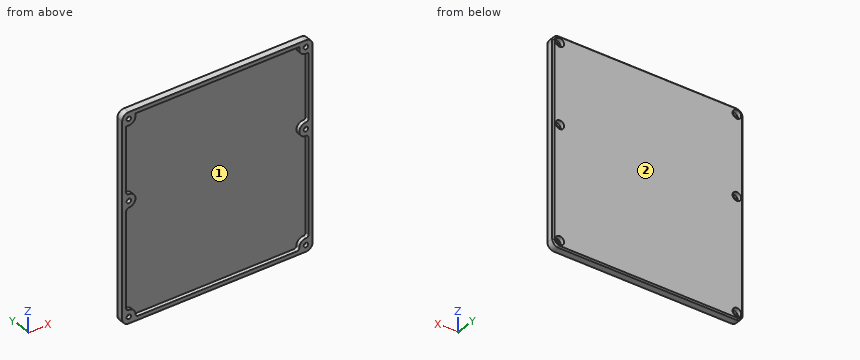
```python
from build123d import *

# Parameters (mm, degrees)
SKETCH_1_W                   = 144
SKETCH_1_H                   = 157
EXTRUDE_1_DEPTH              = 6
FILLET_1_R                   = 5
SHELL_1_T                    = -3
EXTRUDE_2_DEPTH              = 6
HOLE_WIZARD_M3_1_D           = 3.4
HOLE_WIZARD_M3_1_CBORE_D     = 6.5
HOLE_WIZARD_M3_1_CBORE_DEPTH = 3.4
CHAMFER_1_SIZE               = 1
FILLET_4_R                   = 2


with BuildPart() as part:
    # 草图1 → 凸台-拉伸1 (new body)
    with BuildSketch(Plane(origin=(0, 0, 0), x_dir=(1, 0, 0), z_dir=(0, 1, 0))):
        Rectangle(SKETCH_1_W, SKETCH_1_H)
    extrude(amount=EXTRUDE_1_DEPTH)

    # 圆角1
    fillet_1_edges = [part.edges().sort_by_distance(p)[0] for p in [
        (72, 3, 78.5),
        (-72, 3, 78.5),
        (-72, 3, -78.5),
        (72, 3, -78.5),
    ]]
    fillet(fillet_1_edges, radius=FILLET_1_R)

    # 抽壳1
    shell_1_openings = [part.faces().sort_by_distance(p)[0] for p in [
        (0, 0, 0),
    ]]
    offset(amount=SHELL_1_T, openings=shell_1_openings, kind=Kind.INTERSECTION)

    # 草图3 → 凸台-拉伸2 (add)
    with BuildSketch(Plane(origin=(0, 6, 0), x_dir=(1, 0, 0), z_dir=(0, 1, 0))):
        with BuildLine():
            Line((-62, 73.5), (-62, 77.035533906))
            Line((-62, 77.035533906), (-70.535533906, 77.035533906))
            Line((-70.535533906, 77.035533906), (-70.535533906, 68.5))
            Line((-70.535533906, 68.5), (-67, 68.5))
            ThreePointArc((-67, 68.5), (-63.464466094, 69.964466094), (-62, 73.5))
        make_face()
        with BuildLine():
            Line((-67, -7.5), (-72, -7.5))
            Line((-72, -7.5), (-72, -17.5))
            Line((-72, -17.5), (-67, -17.5))
            ThreePointArc((-67, -17.5), (-62, -12.5), (-67, -7.5))
        make_face()
        with BuildLine():
            Line((72, -7.5), (72, -17.5))
            Line((72, -17.5), (67, -17.5))
            ThreePointArc((67, -17.5), (62, -12.5), (67, -7.5))
            Line((67, -7.5), (72, -7.5))
        make_face()
        with BuildLine():
            Line((70.535533906, 68.5), (67, 68.5))
            ThreePointArc((67, 68.5), (63.464466094, 69.964466094), (62, 73.5))
            Line((62, 73.5), (62, 77.035533906))
            Line((62, 77.035533906), (70.535533906, 77.035533906))
            Line((70.535533906, 77.035533906), (70.535533906, 68.5))
        make_face()
        with BuildLine():
            Line((62, -73.5), (62, -77.035533906))
            Line((62, -77.035533906), (70.535533906, -77.035533906))
            Line((70.535533906, -77.035533906), (70.535533906, -68.5))
            Line((70.535533906, -68.5), (67, -68.5))
            ThreePointArc((67, -68.5), (63.464466094, -69.964466094), (62, -73.5))
        make_face()
        with BuildLine():
            Line((-62, -73.5), (-62, -77.035533906))
            Line((-62, -77.035533906), (-70.535533906, -77.035533906))
            Line((-70.535533906, -77.035533906), (-70.535533906, -68.5))
            Line((-70.535533906, -68.5), (-67, -68.5))
            ThreePointArc((-67, -68.5), (-63.464466094, -69.964466094), (-62, -73.5))
        make_face()
    extrude(amount=-EXTRUDE_2_DEPTH)

    # M3 六角凹头螺钉的柱形沉头孔1 (through all)
    with Locations(Plane(origin=(0, 6, 0), x_dir=(-1, 0, 0), z_dir=(0, 1, 0))):
        with Locations((67, 12.5), (67, -73.5), (-67, -73.5), (-67, 12.5), (-67, 73.5), (67, 73.5)):
            CounterBoreHole(HOLE_WIZARD_M3_1_D / 2, HOLE_WIZARD_M3_1_CBORE_D / 2, HOLE_WIZARD_M3_1_CBORE_DEPTH)

    # 倒角1
    chamfer_1_edges = [part.edges().sort_by_distance(p)[0] for p in [
        (72, 6, 0),
        (0, 6, 78.5),
        (0, 6, -78.5),
        (-72, 6, 0),
        (-70.535533906, 6, -77.035533906),
        (70.535533906, 6, -77.035533906),
        (-70.535533906, 6, 77.035533906),
        (70.535533906, 6, 77.035533906),
    ]]
    chamfer(chamfer_1_edges, length=CHAMFER_1_SIZE)

    # 圆角4
    fillet_4_edges = [part.edges().sort_by_distance(p)[0] for p in [
        (69, 1.5, -68.5),
        (62, 1.5, -75.5),
        (69, 1.5, 7.5),
        (69, 1.5, 17.5),
        (-69, 1.5, 17.5),
        (-62, 1.5, -75.5),
        (-69, 1.5, -68.5),
        (-69, 1.5, 7.5),
    ]]
    fillet(fillet_4_edges, radius=FILLET_4_R - 0.0001)  # a hair under: the kernel refuses the full size


solid = part.part
```
Read the model definition and answer for the solid it produces. Units are mm, in the model's axes. Face numbers are marked on the shaded views. Give positions to 0.01 mm unless a question says otherwise; leave off trailing zeros. Loops run counter-clockwise (first coordinate to the right, second up) from the corner with the lowest first, then second, coordinate; pieces in that order, holes last.
Item 1: The part is cut by section B-B (z = -48.5). Write down the section's boundary in (x, y), and give its area (3 significant figures).
Item 2: Find the intervals of material crossed by line 1 along Z through (x, y) = (-67, 4.2); line 2 along X through (y, z) = (2, 73.5); line 3 along Z through (x, y) = (-67, 1), in increasing order.
Item 3: The mould has two halves that part along Z. Classify the marked faces 1 and 2: released by +Z, released by -Z, zero draft, split by the parting line, or undercut.
Item 4: Each of these flat-tipped pins is pushed along its axis until it touches: pin 1 Ø2 at (x, z) = (36, -1) entering from -Y; pin 2 Ø2.5 at (x, z) = (67, 73.5) entering from -Y; pin 3 Ø0.6 at (x, y) = (68.5, 1) entering from -Z. Where does it stop, or does it pass through?
Item 5: The part is cut by section A-A (x = 3.5). Write down the section's boundary in (y, z).
Taken from the geometry:
1. outline: (-72, 0) - (-69, 0) - (-69, 3) - (69, 3) - (69, 0) - (72, 0) - (72, 5) - (71, 6) - (-71, 6) - (-72, 5) - close
1. area: 449 mm2
2. line 1: z = -78.5 to -76.75, -70.25 to 9.25, 15.75 to 70.25, 76.75 to 78.5
2. line 2: x = -72 to -68.7, -65.3 to -62, 62 to 65.3, 68.7 to 72
2. line 3: z = -78.5 to -75.2, -71.8 to -68.5, 7.5 to 10.8, 14.2 to 17.5, 68.5 to 71.8, 75.2 to 78.5
3. face 1: undercut
3. face 2: zero draft
4. pin 1: stops at y = 3
4. pin 2: passes through
4. pin 3: stops at z = -78.35
5. outline: (0, -78.5) - (5, -78.5) - (6, -77.5) - (6, 77.5) - (5, 78.5) - (0, 78.5) - (0, 75.5) - (3, 75.5) - (3, -75.5) - (0, -75.5) - close
